from build123d import *

# Parameters (mm, degrees)
SKETCH2_R           = 1.5
BOSS_EXTRUDE1_DEPTH = 2.5


with BuildPart() as part:
    # Sketch2 → Boss-Extrude1 (new body)
    with BuildSketch(Plane.XY):
        Polygon((0, 0), (106.066017178, 106.066017178), (0, 212.132034356), (-106.066017178, 106.066017178), align=None)
        with Locations((-7.5, 197.132034356)):
            Circle(SKETCH2_R, mode=Mode.SUBTRACT)
        with Locations((7.5, 197.132034356)):
            Circle(SKETCH2_R, mode=Mode.SUBTRACT)
        with Locations((-7.5, 187.132034356)):
            Circle(SKETCH2_R, mode=Mode.SUBTRACT)
        with Locations((7.5, 187.132034356)):
            Circle(SKETCH2_R, mode=Mode.SUBTRACT)
        with Locations((81.066019356, 113.566015)):
            Circle(SKETCH2_R, mode=Mode.SUBTRACT)
        with Locations((81.066019356, 98.566015)):
            Circle(SKETCH2_R, mode=Mode.SUBTRACT)
        with Locations((91.066019356, 98.566015)):
            Circle(SKETCH2_R, mode=Mode.SUBTRACT)
        with Locations((91.066019356, 113.566015)):
            Circle(SKETCH2_R, mode=Mode.SUBTRACT)
        with Locations((7.5, 24.999995644)):
            Circle(SKETCH2_R, mode=Mode.SUBTRACT)
        with Locations((-7.5, 24.999995644)):
            Circle(SKETCH2_R, mode=Mode.SUBTRACT)
        with Locations((-7.5, 14.999995644)):
            Circle(SKETCH2_R, mode=Mode.SUBTRACT)
        with Locations((7.5, 14.999995644)):
            Circle(SKETCH2_R, mode=Mode.SUBTRACT)
        with Locations((-81.066019356, 98.566015)):
            Circle(SKETCH2_R, mode=Mode.SUBTRACT)
        with Locations((-81.066019356, 113.566015)):
            Circle(SKETCH2_R, mode=Mode.SUBTRACT)
        with Locations((-91.066019356, 113.566015)):
            Circle(SKETCH2_R, mode=Mode.SUBTRACT)
        with Locations((-91.066019356, 98.566015)):
            Circle(SKETCH2_R, mode=Mode.SUBTRACT)
    extrude(amount=BOSS_EXTRUDE1_DEPTH)


solid = part.part
The listing builds one solid part. Answer for the finished solid, in the listing's coordinates (mm). Round coordinates to 2 decimals unless told otherwise and drop trailing zeros. Loops run counter-clockwise (first coordinate to the right, second up) from the corner with the lowest first, then second, coordinate; pieces in that order, holes last. Notation, with made-up numbers: M -10.75,28.25 L 44.25,28.25 A18 cw 44.25,53.25 Z; hole C 18,32 d11. An arc over 180 degrees is marked long. Write each question's results on one line, items separated by ' | '. Start each with the question number.
1) Straight lines are drawn through the part: probe 1 along Y at (x, z) = (7.5, 1.15); probe 2 along Y at (x, z) = (90.5, 0.95); probe 3 along X at (y, z) = (64, 1.75). For each, find the intervals that lie inside material, in ascending order.
2) Find section A-A on z = 0.95. Count the separate pieces of the cut face and the enclosed holes in it, plus the area to 3 significant figures.
3) Find section C-C on x = 28. Write down the section's boundary in (y, z), plus the area to 3 significant figures.
4) Each of these flat-tipped pins is pushed along its axis until it touches: pin 1 (5 mm diameter, centred on x = -7.5, y = 15, fed in from -Z); pin 2 (1 mm diameter, centred on y = 117, z = 1.5, fed in from +X); pin 3 (1 mm diameter, centred on x = 30.5, z = 1, fed in from -Y); pin 4 (1.5 mm diameter, centred on x = 32.5, z = 1.5, fed in from -Y). Where does it stop, or does it pass through?
5) Find section B-B on y = 69. Write down the section's boundary in (x, z), plus the area to 3 significant figures.
Final values:
1) probe 1: 7.5 to 13.5, 16.5 to 23.5, 26.5 to 185.63, 188.63 to 195.63, 198.63 to 204.63 | probe 2: 90.5 to 97.18, 99.96 to 112.18, 114.96 to 121.63 | probe 3: -64 to 64
2) separate pieces: 1 | enclosed holes: 16 | area: 22,400 mm²
3) outline: M 28,0 L 184.13,0 L 184.13,2.5 L 28,2.5 Z | area: 390 mm²
4) pin 1: z = 0 | pin 2: x = 95.63 | pin 3: y = 30 | pin 4: y = 31.75
5) outline: M -69,0 L 69,0 L 69,2.5 L -69,2.5 Z | area: 345 mm²
